from build123d import *

# Parameters (mm, degrees)
SKETCH1_W           = 70
SKETCH1_H           = 70
SKETCH1_W_2         = 64
SKETCH1_H_2         = 64
BOSS_EXTRUDE1_DEPTH = 860
FILLET1_R           = 5
SKETCH2_R           = 3
CUT_EXTRUDE1_DEPTH  = 70
LPATTERN1_COUNT     = 9
LPATTERN1_PITCH     = 35
LPATTERN1_COL_COUNT = 9
LPATTERN1_COL_PITCH = 35


with BuildPart() as part:
    # Sketch1 → Boss-Extrude1 (new body)
    with BuildSketch(Plane(origin=(0, 0, 0), x_dir=(1, 0, 0), z_dir=(0, 1, 0))):
        with Locations((35, 35)):
            Rectangle(SKETCH1_W, SKETCH1_H)
        with Locations((35, 35)):
            Rectangle(SKETCH1_W_2, SKETCH1_H_2, mode=Mode.SUBTRACT)
    extrude(amount=BOSS_EXTRUDE1_DEPTH)

    # Fillet1
    fillet1_edges = [part.edges().sort_by_distance(p)[0] for p in [
        (3, 430, -67),
        (3, 430, -3),
        (67, 430, -3),
        (67, 430, -67),
        (0, 430, 0),
        (0, 430, -70),
        (70, 430, -70),
        (70, 430, 0),
    ]]
    fillet(fillet1_edges, radius=FILLET1_R)

    # Sketch2 → Cut-Extrude1 (cut)
    with BuildSketch(Plane(origin=(0, 0, -70), x_dir=(-1, 0, 0), z_dir=(0, 0, -1))):
        with Locations((-35, 430)):
            Circle(SKETCH2_R)
    cut_extrude1 = extrude(amount=-CUT_EXTRUDE1_DEPTH, mode=Mode.SUBTRACT)

    # LPattern1: Cut-Extrude1 ×9
    with Locations(*[(0, -i * LPATTERN1_PITCH, 0) for i in range(1, LPATTERN1_COUNT)]):
        add(cut_extrude1, mode=Mode.SUBTRACT)

    # LPattern1 col: Cut-Extrude1 ×9
    with Locations(*[(0, i * LPATTERN1_COL_PITCH, 0) for i in range(1, LPATTERN1_COL_COUNT)]):
        add(cut_extrude1, mode=Mode.SUBTRACT)


solid = part.part
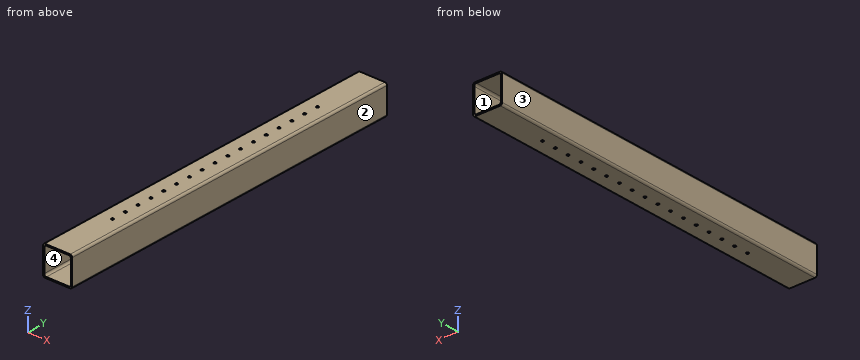
Verification items for the finished model (mm, model axes). Face numbers are marked on the shaded views. Round coordinates to 2 decimals unless told otherwise and drop trailing zeros. Loops run counter-clockwise (first coordinate to the right, second up) from the corner with the lowest first, then second, coordinate; pieces in that order, holes last. Notation, with made-up numbers: (-32, 0) - (25, 0) arc R23 ccw to (25, 15) - close; hole circle Ø11 at (15.25, 67.25). An arc over 180 degrees is marked (long way). Answer in a Markdown table with one row per item. Add a question column.
Q1. Material ranges on line 1 (Z direction, x = 42, y = 173); line 2 (X direction, y = 400, z = -43); line 3 (X direction, y = 399.5, z = -4), recorded low to high.
Q2. Section check C-C on z = -17.5. Enter the section's corners in (x, y).
Q3. Section check A-A on y = 446. Enter the section's corners in (x, z).
Q4. Section check B-B on x = 53.5. Enter the section's corners in (y, z), plus the area to 3 significant figures.
Q5. Gauge pin test, flat end, axial feed: pin 1 (8 mm diameter, centred on x = 35, y = 395, fed in from -Z). Record the tip position at first contact, or that the pin passes through.
Q6. Release check for a two-part mould opening along X. For the marked faces 1, 2, 3 and 4 record: pulls with the +X half, pulls with the -X half, needs draft (parallel to the pull), parting line crosses it, or undercut.
Found:
| question | item | result |
|---|---|---|
| 1 | line 1 | z = -70 to -67, -3 to 0 |
| 1 | line 2 | x = 0 to 3, 67 to 70 |
| 1 | line 3 | x = 0.1 to 5, 65 to 69.9 |
| 2 | outline | (0, 0) - (3, 0) - (3, 860) - (0, 860) - close; (67, 0) - (70, 0) - (70, 860) - (67, 860) - close |
| 3 | outline | (0, -65) arc R5 ccw to (5, -70) - (65, -70) arc R5 ccw to (70, -65) - (70, -5) arc R5 ccw to (65, 0) - (5, 0) arc R5 ccw to (0, -5) - close; hole (3, -62) arc R5 ccw to (8, -67) - (62, -67) arc R5 ccw to (67, -62) - (67, -8) arc R5 ccw to (62, -3) - (8, -3) arc R5 ccw to (3, -8) - close |
| 4 | outline | (0, -70) - (860, -70) - (860, -67) - (0, -67) - close; (0, -3) - (860, -3) - (860, 0) - (0, 0) - close |
| 4 | area | 5,160 mm² |
| 5 | pin 1 | stops at z = -70 |
| 6 | face 1 | undercut |
| 6 | face 2 | pulls with the +X half |
| 6 | face 3 | pulls with the -X half |
| 6 | face 4 | undercut |
